Input: part model. Units: mm. Frame: model coordinates. A direction names the side the tool comes from. Coordinates: 2 decimals unless noted, no trailing zeros. Loops run counter-clockwise (first coordinate to the right, second up) from the corner with the lowest first, then second, coordinate; pieces in that order, holes last. Notation, with made-up numbers: (27, 89.5) - (39, 89.5) arc R22 ccw to (39, 111.5) - close; hole circle Ø10 at (61.5, 76.5). An arc over 180 degrees is marked (long way). Use a Markdown table: item, result. Add a question column.
1. Contact query for a flat-ended pin moving along its axis: P1, Ø4, axis at x = 71.5, y = 7.5, coming from the +Z side. Output: stop coordinate, or through.
2. Ray query, L1, parallel to X at y = 10, z = 48.5; L2, parallel to Y at x = 74.5, z = 53. Return the intervals inside material, ascending. Write a range as [from, to].
3. Access query for faces 1 (the face through (69, 6, 43)), 2 (the face through (73, 6, 29)), 3 (the face through (45, 0, 30)). Directions: +Z, -Z, +X, -X, +Y, -Y. A direction counts if a zero-diameter tool reaches every point of the face in a straight line with its end or side. Return the directions, or none.
4. Section query A-A on z = 40.5. Return the cut outline in (x, y).
5. Draft query along Z for faces 4 (the face through (73, 6, 26.015)), 5 (the face through (73, 6, 31)), 6 (the face through (92.001, 32, 30)). Return one class per face: released by +Z, released by -Z, zero draft, split by the parting line, or undercut.
```python
from build123d import *

# Parameters (mm, degrees)
BOSS_EXTRUDE1_DEPTH = 60
SKETCH1_6_W         = 8.001
SKETCH1_6_H         = 12.31
BOSS_EXTRUDE3_DEPTH = 26.01546
SKETCH2_W           = 2
SKETCH2_H           = 2
BOSS_EXTRUDE4_DEPTH = 12.31


with BuildPart() as part:
    # Sketch1 → Boss-Extrude1 (new body)
    with BuildSketch(Plane.XY):
        Polygon((77.001, 12.31), (77.001, 0), (92.001, 0), (92.001, 65.01), (0, 65.01), (0, 0), (69, 0), (69, 12.31), align=None)
    extrude(amount=BOSS_EXTRUDE1_DEPTH)

    # Sketch1<6> → Boss-Extrude3 (add)
    with BuildSketch(Plane.XY):
        with Locations((73.0005, 6.155)):
            Rectangle(SKETCH1_6_W, SKETCH1_6_H)
    extrude(amount=BOSS_EXTRUDE3_DEPTH)

    # Sketch2 → Boss-Extrude4 (add)
    with BuildSketch(Plane.XZ):
        with Locations((73.0005, 30.00046)):
            Rectangle(SKETCH2_W, SKETCH2_H)
    extrude(amount=-BOSS_EXTRUDE4_DEPTH)


solid = part.part
```
Resolved:
| question | item | result |
|---|---|---|
| 1 | P1 | z = 31 |
| 2 | L1 | [0, 69], [77, 92] |
| 2 | L2 | [12.31, 65.01] |
| 3 | face 1 | +Z, -Y |
| 3 | face 2 | -Y |
| 3 | face 3 | +Z, -Z, +X, -X, -Y |
| 4 | outline | (0, 0) - (69, 0) - (69, 12.31) - (77, 12.31) - (77, 0) - (92, 0) - (92, 65.01) - (0, 65.01) - close |
| 5 | face 4 | undercut |
| 5 | face 5 | released by +Z |
| 5 | face 6 | zero draft |
